Geometry check sheet. Reference: the model listing, model coordinates, mm. Give positions to 0.01 mm unless a question says otherwise; leave off trailing zeros. Write each loop counter-clockwise with the first axis right and the second up, starting at its lowest first coordinate (ties: lowest second). Pieces come first, ordered by that corner, then holes. Notation, with made-up numbers: (38.5, 14.5) - (73.5, 14.5) arc R17 cw to (73.5, 27.5) - close; hole circle Ø3 at (66.25, 36.25). An arc over 180 degrees is marked (long way). Use a Markdown table: item, result.
```python
from build123d import *

# Parameters (mm, degrees)
F3_DEPTH = 50.8


with BuildPart() as f1:
    # F0 (on Front) → F1 (revolve)
    with BuildSketch(Plane.XZ):
        Polygon((-45.2943, -32.033801), (0, -32.033801), (0, 43.953352), (-15.49542, 43.953352), (-28.308939, 31.735811), (-38.142569, 14.452458), (-45.2943, -9.982626), align=None)
    revolve(axis=Axis((0, 0, 5.959775), (0, 0, -1)))

    # F2 (on Front) → F3 (join)
    with BuildSketch(Plane.XZ):
        Polygon((6.767772, 19.607749), (-7.021107, 19.607749), (0, 7.457786), align=None)
    extrude(amount=F3_DEPTH)


solid = f1.part
```
1) Depth check by flat-ended pin: P1, Ø6, axis at y = 35, z = 15.5, coming from the -X side; P2, Ø3, axis at x = 15, z = 5.5, coming from the +Y side; P3, Ø4, axis at y = 25, z = 27.5, coming from the -X side. Enter the tip coordinate at first touch or a pass-through.
Working result:
| item | result |
|---|---|
| P1 | stops at x = -20.46 |
| P2 | stops at y = 38.64 |
| P3 | stops at x = -20.94 |
2) Section check A-A on y = 0. Record the boundary of the cut face in (x, z), then the cut area to 3 significant figures.
Working result:
| item | result |
|---|---|
| outline | (-45.29, -32.03) - (45.29, -32.03) - (45.29, -9.98) - (38.14, 14.45) - (28.31, 31.74) - (15.5, 43.95) - (-15.5, 43.95) - (-28.31, 31.74) - (-38.14, 14.45) - (-45.29, -9.98) - close |
| area | 5,720 mm² |
3) Section check B-B on z = -13. Record the boundary of the cut face in (x, y), then the cut area to 3 significant figures.
Working result:
| item | result |
|---|---|
| outline | circle Ø90.59 at (0, 0) |
| area | 6,450 mm² |
4) Mould release check, pull along Z, two halves, no side actions. Record for faces 1 (the conical face through (-15.54, 4.9, 43.19)), 2 (the flat face through (3.34, -44.37, 13.45)), 3 (the flat face through (-3.56, -44.35, 13.62)), 4 (the flat face through (0, -50.8, 15)): pulls with the +Z half, pulls with the -Z half, needs draft (parallel to the pull), parting line crosses it, or undercut.
Working result:
| item | result |
|---|---|
| face 1 | pulls with the +Z half |
| face 2 | undercut |
| face 3 | undercut |
| face 4 | needs draft |
5) Material ranges on L1, parallel to X at y = 0.5, z = 21; L2, parallel to X at y = -30.5, z = 19; L3, parallel to Z at x = -7.5, y = -28, recorded low to high. Write a range as from..to.
Working result:
| item | result |
|---|---|
| L1 | x = -34.41..34.41 |
| L2 | x = -18.27..18.27 |
| L3 | z = -32.03..30.54 |
6) Section check C-C on z = 33. Record the boundary of the cut face in (x, y).
Working result:
| item | result |
|---|---|
| outline | circle Ø53.97 at (0, 0) |
